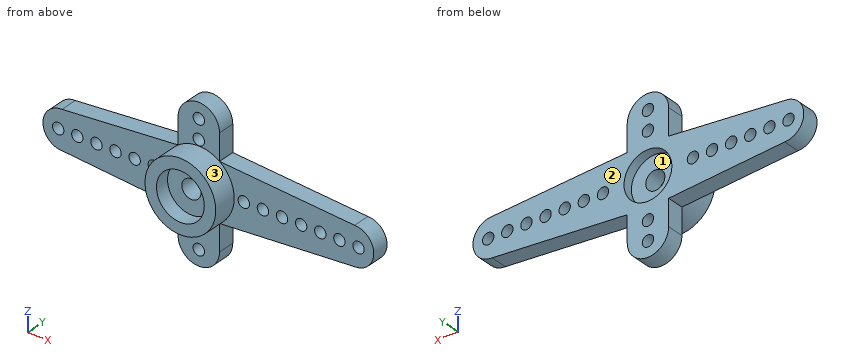
```python
from build123d import *

# Parameters (mm, degrees)
CROQUIS1_R              = 3.7
SALIENTE_EXTRUIR2_DEPTH = 4.3
CROQUIS2_R              = 2.5
CORTAR_EXTRUIR1_DEPTH   = 1.5
CROQUIS3_R              = 2.5
CORTAR_EXTRUIR2_DEPTH   = 1
CROQUIS4_R              = 1
CORTAR_EXTRUIR3_DEPTH   = 1.8
SALIENTE_EXTRUIR3_DEPTH = 1.8
CROQUIS6_R              = 0.595
CORTAR_EXTRUIR4_DEPTH   = 1.8
CROQUIS7_R              = 0.595
SALIENTE_EXTRUIR4_DEPTH = 1.8


with BuildPart() as part:
    # Croquis1 → Saliente-Extruir2 (new body)
    with BuildSketch(Plane(origin=(0, 0, 0), x_dir=(1, 0, 0), z_dir=(0, 1, 0))):
        Circle(CROQUIS1_R)
    extrude(amount=SALIENTE_EXTRUIR2_DEPTH)

    # Croquis2 → Cortar-Extruir1 (cut)
    with BuildSketch(Plane.XZ):
        Circle(CROQUIS2_R)
    extrude(amount=-CORTAR_EXTRUIR1_DEPTH, mode=Mode.SUBTRACT)

    # Croquis3 → Cortar-Extruir2 (cut)
    with BuildSketch(Plane(origin=(0, 4.3, 0), x_dir=(1, 0, 0), z_dir=(0, 1, 0))):
        Circle(CROQUIS3_R)
    extrude(amount=-CORTAR_EXTRUIR2_DEPTH, mode=Mode.SUBTRACT)

    # Croquis4 → Cortar-Extruir3 (cut)
    with BuildSketch(Plane(origin=(0, 3.3, 0), x_dir=(1, 0, 0), z_dir=(0, 1, 0))):
        Circle(CROQUIS4_R)
    extrude(amount=-CORTAR_EXTRUIR3_DEPTH, mode=Mode.SUBTRACT)

    # Croquis5 → Saliente-Extruir3 (add)
    with BuildSketch(Plane(origin=(0, 4.3, 0), x_dir=(1, 0, 0), z_dir=(0, 1, 0))):
        with BuildLine():
            Line((-2.16564, 3.000000565), (-3.120237459, 0))
            Line((-3.120237459, 0), (-2.16564, -3.000000565))
            Line((-2.16564, -3.000000565), (-14.3, -2))
            ThreePointArc((-14.3, -2), (-16.3, 0), (-14.3, 2))
            Line((-14.3, 2), (-2.16564, 3.000000565))
        make_face()
        with BuildLine():
            Line((3.120237459, 0), (2.16564, -3.000000565))
            Line((2.16564, -3.000000565), (16.3, -2))
            ThreePointArc((16.3, -2), (18.3, 0), (16.3, 2))
            Line((16.3, 2), (2.16564, 3.000000565))
            Line((2.16564, 3.000000565), (3.120237459, 0))
        make_face()
    extrude(amount=-SALIENTE_EXTRUIR3_DEPTH)

    # Croquis6 → Cortar-Extruir4 (cut)
    with BuildSketch(Plane(origin=(0, 4.3, 0), x_dir=(1, 0, 0), z_dir=(0, 1, 0))):
        with Locations((-14.705, 0)):
            Circle(CROQUIS6_R)
        with Locations((-12.705, 0)):
            Circle(CROQUIS6_R)
        with Locations((-10.705, 0)):
            Circle(CROQUIS6_R)
        with Locations((-8.705, 0)):
            Circle(CROQUIS6_R)
        with Locations((-6.705, 0)):
            Circle(CROQUIS6_R)
        with Locations((-4.705, 0)):
            Circle(CROQUIS6_R)
        with Locations((14.705, 0)):
            Circle(CROQUIS6_R)
        with Locations((12.705, 0)):
            Circle(CROQUIS6_R)
        with Locations((10.705, 0)):
            Circle(CROQUIS6_R)
        with Locations((8.705, 0)):
            Circle(CROQUIS6_R)
        with Locations((6.705, 0)):
            Circle(CROQUIS6_R)
        with Locations((4.705, 0)):
            Circle(CROQUIS6_R)
        with Locations((16.705, 0)):
            Circle(CROQUIS6_R)
    extrude(amount=-CORTAR_EXTRUIR4_DEPTH, mode=Mode.SUBTRACT)

    # Croquis7 → Saliente-Extruir4 (add)
    with BuildSketch(Plane(origin=(0, 4.3, 0), x_dir=(1, 0, 0), z_dir=(0, 1, 0))):
        with BuildLine():
            Line((-2.16564, 3.000000565), (2.16564, 3.000000565))
            Line((2.16564, 3.000000565), (2.16564, 5.750000565))
            ThreePointArc((2.16564, 5.750000565), (0, 7.915640565), (-2.16564, 5.750000565))
            Line((-2.16564, 5.750000565), (-2.16564, 3.000000565))
        make_face()
        with Locations((0, 6.320640565)):
            Circle(CROQUIS7_R, mode=Mode.SUBTRACT)
        with Locations((0, 4.320640565)):
            Circle(CROQUIS7_R, mode=Mode.SUBTRACT)
        with BuildLine():
            Line((2.16564, -3.000000565), (2.16564, -5.750000565))
            ThreePointArc((2.16564, -5.750000565), (0, -7.915640565), (-2.16564, -5.750000565))
            Line((-2.16564, -5.750000565), (-2.16564, -3.000000565))
            Line((-2.16564, -3.000000565), (2.16564, -3.000000565))
        make_face()
        with Locations((0, -4.320640565)):
            Circle(CROQUIS7_R, mode=Mode.SUBTRACT)
        with Locations((0, -6.320640565)):
            Circle(CROQUIS7_R, mode=Mode.SUBTRACT)
    extrude(amount=-SALIENTE_EXTRUIR4_DEPTH)


solid = part.part
```
Read the model definition and answer for the solid it produces. Units are mm, in the model's axes. Face numbers are marked on the shaded views. A direction names the side the tool comes from. Coordinates: 2 decimals unless noted, no trailing zeros. Loops run counter-clockwise (first coordinate to the right, second up) from the corner with the lowest first, then second, coordinate; pieces in that order, holes last.
(1) Consider line 1 along Z through (x, y) = (0, 3.85); line 2 along Y through (x, z) = (12, -0.75); line 3 along X through (y, z) = (2.9, 5.5). Determine where each line is inside the solid, lowest interval first.
Solution:
line 1: z = -7.92 to -6.92, -5.73 to -4.92, -3.73 to -2.5, 2.5 to 3.73, 4.92 to 5.73, 6.92 to 7.92
line 2: y = 2.5 to 4.3
line 3: x = -2.17 to 2.17
(2) A tool of negligible diameter and unlimited length cuts with its end or side. For the marked faces 1, 2 and 3, from which of +Z, -Z, +X, -X, +Y, -Y can it reach the whole face along a straight path? Write none if from no direction.
Solution:
face 1: +Y
face 2: +Z, -Z, +X, -X, +Y
face 3: -Y
(3) The part is cut by section B-B (y = 0.8). Determine the outline of the cut face in (x, z).
Solution:
outline: circle Ø7.4 at (0, 0); hole circle Ø5 at (0, 0)
(4) Flat-ended cylindrical pins translate along their axes: pin 1 Ø1 at (x, z) = (-12.705, 0) entering from +Y; pin 2 Ø1.4 at (y, z) = (3, -5) entering from +X; pin 3 Ø0.5 at (y, z) = (3.5, 4.5) entering from -X; pin 4 Ø3.5 at (x, z) = (0.5, 5.5) entering from -Y. Find the tip coordinate at first contact, or state that the pin passes through.
Solution:
pin 1: passes through
pin 2: stops at x = 2.17
pin 3: stops at x = -2.17
pin 4: stops at y = 2.5
(5) The part is cut by section A-A (z = 0). Count the separate pieces of the cut face and the enclosed holes in it, and give its area (3 significant figures).
Solution:
separate pieces: 15
enclosed holes: 0
area: 36.8 mm2
